Verification items for the finished model (mm, model axes). Give positions to 0.01 mm unless a question says otherwise; leave off trailing zeros. Order: outer loops, then holes, each group sorted by start corner. A loop starts at its lowest first (then second) coordinate and runs counter-clockwise, first axis right, second up. Notation, with made-up numbers: (12.5, 68.25) -> (43.5, 68.25) arc R12 ccw to (43.5, 82.25) -> close; hole circle Ø9 at (-2, 23.5). An arc over 180 degrees is marked (long way). Write each question's results on one line, items separated by ' | '. Start each with the question number.
1. Cross-section at B-B, the plane y = -9.25. Enter the section's corners in (x, z), then the cut area to 3 significant figures.
2. Material ranges on L1, parallel to Z at x = 0, y = -5.5; L2, parallel to X at y = -14, z = 4.5; L3, parallel to Z at x = 120, y = -10.5, recorded low to high. Write a range as from..to.
3. Depth check by flat-ended pin: pin 1 Ø2 at (y, z) = (-21, -104) entering from -X; pin 2 Ø12 at (y, z) = (-11.5, 101) entering from +X; pin 3 Ø10 at (y, z) = (-17.5, -65) entering from +X. Enter the tip coordinate at first touch or a pass-through.
4. Cross-section at A-A, the plane z = 0. Enter the section's corners in (x, y), then the cut area to 3 significant figures.
from build123d import *

# Parameters (mm, degrees)
F0_R     = 152.4
F1_DEPTH = 25.4
F2_R     = 5.08
F3_R     = 6.35
F4_DEPTH = 25.4


with BuildPart() as f1:
    # F0 (on Front) → F1 (new body)
    with BuildSketch(Plane.XZ):
        with Locations((2.800982, 0)):
            Circle(F0_R)
    extrude(amount=F1_DEPTH)

    # F2
    f2_edges = [f1.edges().sort_by_distance(p)[0] for p in [
        (-149.599018, -25.4, 0),
        (-149.599018, 0, 0),
    ]]
    fillet(f2_edges, radius=F2_R)

    # F3 (on face) → F4 (cut)
    with BuildSketch(Plane.XZ.offset(25.4)):
        Circle(F3_R)
    extrude(amount=-F4_DEPTH, mode=Mode.SUBTRACT)


solid = f1.part
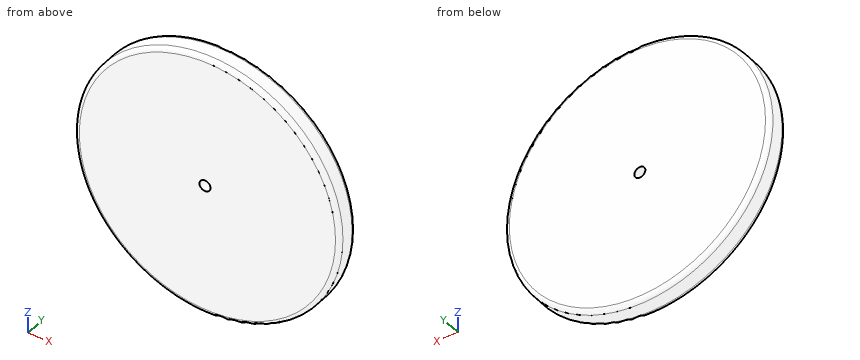
Results below:
1) outline: circle Ø304.8 at (2.8, 0); hole circle Ø12.7 at (0, 0) | area: 72,800 mm²
2) L1: z = -152.37..-6.35, 6.35..152.37 | L2: x = -149.53..-4.48, 4.48..155.13 | L3: z = -97.42..97.42
3) pin 1: stops at x = -109.48 | pin 2: stops at x = 121.97 | pin 3: stops at x = 142.89
4) outline: (-149.6, -20.32) arc R5.08 ccw to (-144.52, -25.4) -> (-6.35, -25.4) -> (-6.35, 0) -> (-144.52, 0) arc R5.08 ccw to (-149.6, -5.08) -> close; (6.35, -25.4) -> (150.12, -25.4) arc R5.08 ccw to (155.2, -20.32) -> (155.2, -5.08) arc R5.08 ccw to (150.12, 0) -> (6.35, 0) -> close | area: 7,400 mm²
